Could you check a few things on this model? Use its own coordinates, in mm. A direction names the side the tool comes from. Round coordinates to 2 decimals unless told otherwise and drop trailing zeros. Write each loop counter-clockwise with the first axis right and the second up, starting at its lowest first coordinate (ties: lowest second). Pieces come first, ordered by that corner, then holes. Notation, with made-up numbers: (88, 9) -> (138, 9) arc R18 ccw to (138, 17) -> close; hole circle Ø8 at (-39, -30.5). An arc over 180 degrees is marked (long way). Answer as CSV lines item,"result". Start each with the question number.
Q1. If we mould it in two halves opening along Z, with no side actions, what happens to faces 4 (the flat face through (0, 20, 99)), 5 (the cylindrical face through (2.6, 4.72, 97.47)), 6 (the flat face through (0, 0, -1.5))? For each: pulls with the +Z half, pulls with the -Z half, needs draft (parallel to the pull), parting line crosses it, or undercut.
Q2. Will these pins go through, and if not, where does the flat tip stop? pin 1 Ø12 at (x, y) = (-5.5, 7) entering from +Z (3 decimals); pin 2 Ø1.5 at (y, z) = (-4, 11.5) entering from -X; pin 3 Ø10 at (x, y) = (-10.5, -9.5) entering from +Z.
Q3. Imagine slicing it at B-B on x = 0. Please give me the cut outline in (y, z).
Q4. Imagine slicing it at A-A on x = -13.5. Please give me the cut outline in (y, z), and give its area (3 significant figures).
Q5. For faces 1 (the cylindrical face through (-14.985, 0.66, -0.74)), 2 (the cylindrical face through (-1.08, 4.88, 48.26)), 3 (the cylindrical face through (-14.2, 0.28, 102.83)), which set-ups out of +Z, -Z, +X, -X, +Y, -Y let a thin tool reach every point of the face, with its end or its side?
Q6. Imagine slicing it at C-C on z = 37. Please give me the cut outline in (x, y), and give its area (3 significant figures).
Q7. If I drill on line 1 (Z direction, x = -3, y = -11); line 2 (Z direction, x = 5, y = 17); line 3 (Z direction, x = -9, y = -5), over which ranges is the centre line in solid material (lowest first)? Write a range as [from, to].
Q8. Imagine slicing it at D-D on x = 7. Please give me the cut outline in (y, z), and give its area (3 significant figures).
Solid Edge part; units mm, degrees
sketch "Sketch1" plane through (0, 0, 0) normal (0, 0, 1) x (1, 0, 0)
  circle A0 centre (0, 0) radius 5
extrude "Protrusion1" add sketch "Sketch1" along normal blind 100
sketch "Sketch2" plane through (0, 0, 0) normal (0, 0, -1) x (1, 0, 0)
  circle A0 centre (0, 0) radius 15
extrude "ExtrudedProtrusion_2" add sketch "Sketch2" along normal blind 1.5
sketch "Sketch3" plane through (0, 0, 0) normal (0, -1, 0) x (1, 0, 0)
  arc A0 (18.9646, 112.9883) -> (-18.9764, 112.9719) centre (-0.0086, 119.3141) cw
  line L0 (-18.9764, 112.9719) -> (-17.3687, 108.1499)
  arc A1 (-17.3687, 108.1499) -> (-10.5859, 100.0237) centre (-3.616, 112.7352) ccw
  arc A2 (10.5838, 100.032) -> (-10.5859, 100.0237) centre (-0.0086, 119.3141) cw
  arc A3 (10.5838, 100.032) -> (17.3613, 108.1655) centre (3.6032, 112.7393) ccw
  line L1 (18.9646, 112.9883) -> (17.3613, 108.1655)
extrude "ExtrudedProtrusion_3" add sketch "Sketch3" along normal mid plane 40
sketch "Sketch4" plane through (-0.0059, -20, 105.1512) normal (0, -1, 0) x (0.3154721, 0, 0.9489349)
  arc A0 (13.4215, -15.5294) -> (1.4367, 20.469) centre (13.4388, 4.4706) cw
  line L0 (1.4367, 20.469) -> (5.9095, 22.7728)
  line L1 (5.9095, 22.7728) -> (18.5638, -15.5294)
  line L2 (18.5638, -15.5294) -> (13.4215, -15.5294)
extrude "ExtrudedCutout_1" cut sketch "Sketch4" against normal blind 62.9052
fillet "Round_1" radius 0.5 2 edges at (18.9646, 0, 112.9883) (-18.9764, 0, 112.9719)
Checks:
1,face 4,"needs draft"
1,face 5,"undercut"
1,face 6,"pulls with the -Z half"
2,pin 1,"z = 102.945"
2,pin 2,"x = -3.8"
2,pin 3,"z = 106.66"
3,outline,"(-20, 97.31) -> (-5, 97.31) -> (-5, 0) -> (-15, 0) -> (-15, -1.5) -> (15, -1.5) -> (15, 0) -> (5, 0) -> (5, 97.31) -> (20, 97.31) -> (20, 99.31) -> (-5, 99.31) -> (-20, 99.31) -> close"
4,outline,"(-20, 102.13) -> (20, 102.13) -> (20, 104.55) -> (-20, 104.55) -> close; (-6.54, -1.5) -> (6.54, -1.5) -> (6.54, 0) -> (-6.54, 0) -> close"
4,area,"116 mm^2"
5,face 1,"-Z"
5,face 2,"none"
5,face 3,"-X, +Y, -Y"
6,outline,"circle Ø10 at (0, 0)"
6,area,"78.5 mm^2"
7,line 1,"[-1.5, 0], [97.52, 99.54]"
7,line 2,"[97.89, 99.95]"
7,line 3,"[-1.5, 0], [99.24, 101.45]"
8,outline,"(-20, 98.46) -> (20, 98.46) -> (20, 100.58) -> (-20, 100.58) -> close; (-13.27, -1.5) -> (13.27, -1.5) -> (13.27, 0) -> (-13.27, 0) -> close"
8,area,"125 mm^2"
